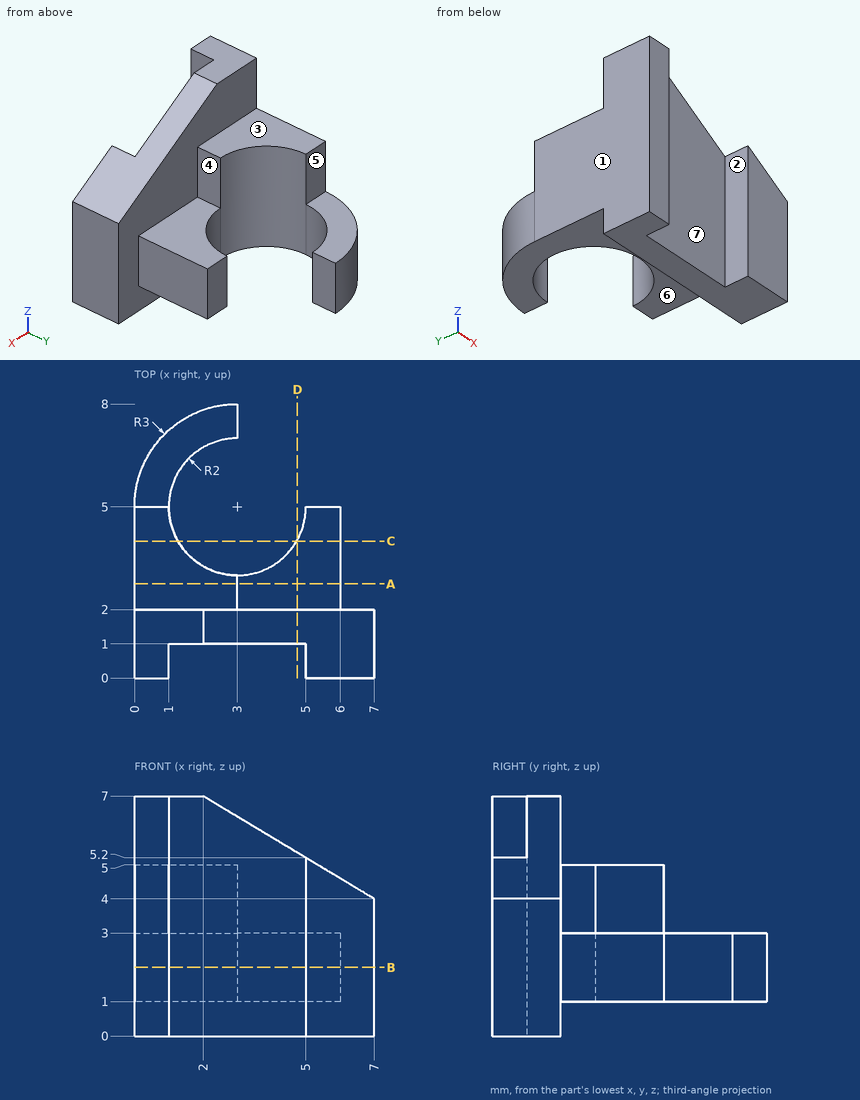
Verification items for this drawing (mm, ordinates from the low corner). A direction names the side the tool comes from. Coordinates: 2 decimals unless noted, no trailing zeros. Loops run counter-clockwise (first coordinate to the right, second up) from the corner with the lowest first, then second, coordinate; pieces in that order, holes last.
Item 1: Thickness scan on line 1 (Y direction, x = 5.5, z = 3.75); line 2 (X direction, y = 4, z = 2.25); line 3 (Z direction, x = 5.75, y = 3). Record the ranges inside material, lowest first.
Item 2: Sectioned sample at B-B, the plane z = 2. Record the boundary of the cut face in (x, y).
Item 3: Access from +Z, -Z, +X, -X, +Y, -Y to the whole of each face (thin tool, end or side, straight path). Record for the marked faces 4, 5, 6 and 7.
Item 4: Sectioned sample at D-D, the plane x = 4.75. Record the boundary of the cut face in (y, z), then the cut area to 3 significant figures.
Item 5: Sectioned sample at A-A, the plane y = 2.75. Record the boundary of the cut face in (x, z).
Item 6: Release check for a two-part mould opening along X. For the marked faces 1, 2 and 3 record: released by +X, released by -X, zero draft, split by the parting line, or undercut.
Item 7: Go/stop test with flat-tipped pins: pin 1 Ø2.5 at (x, y) = (1.5, 6.5) entering from +Z; pin 2 Ø1.1 at (x, z) = (5.5, 2) entering from +Y; pin 3 Ø1 at (x, z) = (2, 6.5) entering from +Y. Record where each tip stops, or that it passes through.
Item 8: Sectioned sample at C-C, the plane y = 4. Record the boundary of the cut face in (x, z), then the cut area to 3 significant figures.
Check result:
1. line 1: y = 0 to 2
1. line 2: x = 0 to 1.27, 4.73 to 6
1. line 3: z = 1 to 3
2. outline: (0, 0) - (1, 0) - (1, 1) - (5, 1) - (5, 0) - (7, 0) - (7, 2) - (6, 2) - (6, 5) - (5, 5) arc R2 cw (long way) to (3, 7) - (3, 8) arc R3 ccw to (0, 5) - close
3. face 4: +Z, +X, +Y
3. face 5: +Z, +X, -X, +Y
3. face 6: -Z, +X, -X, +Y
3. face 7: +Z, -Z, -Y
4. outline: (1, 0) - (2, 0) - (2, 1) - (4.03, 1) - (4.03, 3) - (2, 3) - (2, 5.35) - (1, 5.35) - close
4. area: 9.41 mm2
5. outline: (0, 1) - (6, 1) - (6, 3) - (3, 3) - (3, 5) - (0, 5) - close
6. face 1: released by -X
6. face 2: undercut
6. face 3: zero draft
7. pin 1: stops at z = 3
7. pin 2: stops at y = 5
7. pin 3: stops at y = 2
8. outline: (0, 1) - (1.27, 1) - (1.27, 5) - (0, 5) - close; (4.73, 1) - (6, 1) - (6, 3) - (4.73, 3) - close
8. area: 7.61 mm2
